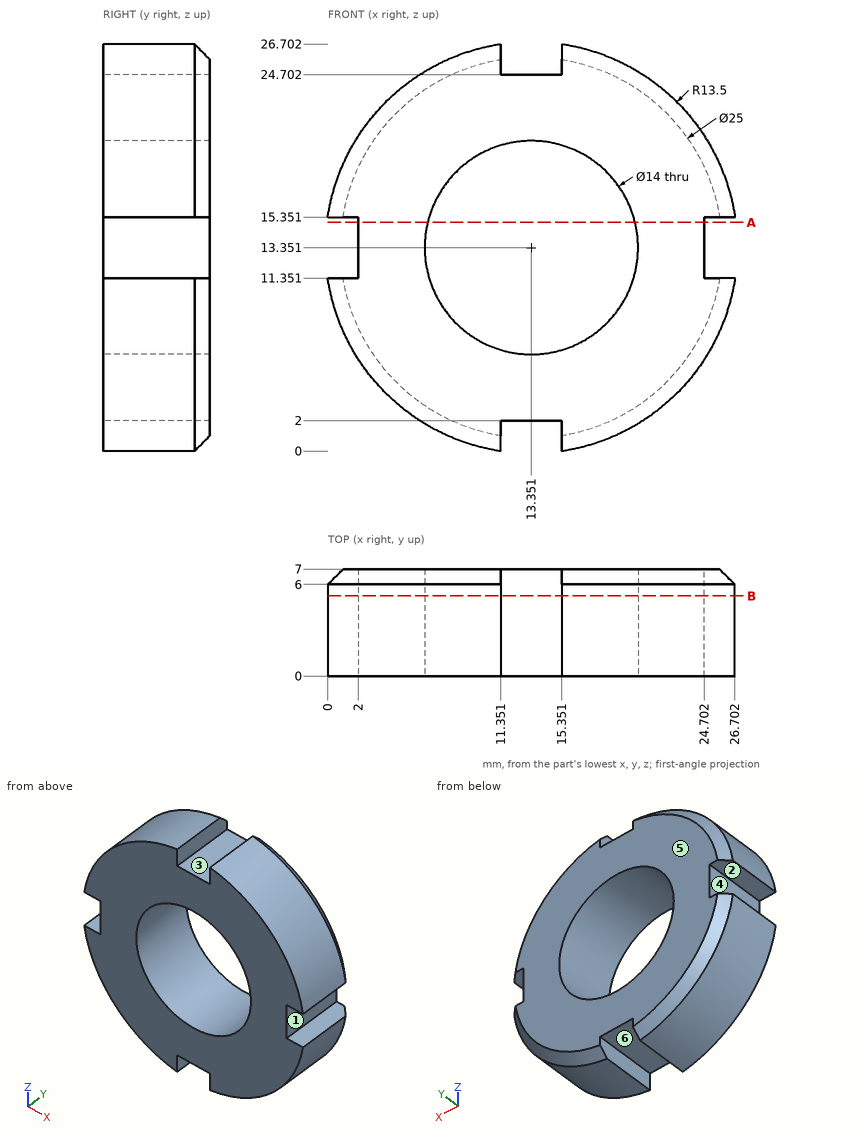
Check sheet for the drawn part. Datum: minimum x, y, z corner. Units: mm. A direction names the side the tool comes from. Round coordinates to 2 decimals unless told otherwise and drop trailing zeros. Loops run counter-clockwise (first coordinate to the right, second up) from the corner with the lowest first, then second, coordinate; pieces in that order, holes last. Notation, with made-up numbers: (70, -12) -> (114, -12) arc R13 cw to (114, 8) -> close; hole circle Ø5 at (84.5, 85.25). An arc over 180 degrees is marked (long way). Put each result on its own line as item: value. Start each with the question number.
1. Draft check along Z on the marked faces 4, 5 and 6. Enter one of: +Z half, -Z half, draft (parallel to the pull), parting line (faces both ways), or undercut.
2. Scan lines: probe 1 along X at (y, z) = (2.75, 12.5); probe 2 along Z at (x, y) = (11.75, 2); probe 3 along X at (y, z) = (2.5, 10) (1 decimal). Record each from-to range of solid material in increasing order.
3. Access from +Z, -Z, +X, -X, +Y, -Y to the whole of each face (thin tool, end or side, straight path). Record for the marked faces 1, 2 and 3.
4. Section check A-A (z = 15). Enter the section's corners in (x, y), plus the area to 3 significant figures.
5. Gauge pin test, flat ends, axial feed: pin 1 (5 mm diameter, centred on x = 9, z = 12.5, fed in from +Y); pin 2 (0.6 mm diameter, centred on y = 5, z = 25.5, fed in from +X); pin 3 (1.2 mm diameter, centred on y = 4.5, z = 14, fed in from +X); pin 4 (1 mm diameter, centred on y = 5, z = 25.5, fed in from -X). Record the tip position at first contact, or that the pin passes through.
6. Section check B-B (y = 5.25). Enter the section's corners in (x, z).
Findings:
1. face 4: undercut
1. face 5: draft
1. face 6: -Z half
2. probe 1: x = 2 to 6.4, 20.3 to 24.7
2. probe 2: z = 2 to 6.54, 20.17 to 24.7
2. probe 3: x = 0.3 to 7.2, 19.5 to 26.4
3. face 1: +X, +Y, -Y
3. face 2: -X, +Y, -Y
3. face 3: +Z, +Y, -Y
4. outline: (2, 0) -> (6.55, 0) -> (6.55, 7) -> (2, 7) -> close; (20.15, 0) -> (24.7, 0) -> (24.7, 7) -> (20.15, 7) -> close
4. area: 63.7 mm^2
5. pin 1: passes through
5. pin 2: stops at x = 19.82
5. pin 3: stops at x = 24.7
5. pin 4: stops at x = 6.53
6. outline: (0, 11.35) arc R13.5 ccw to (11.35, 0) -> (11.35, 2) -> (15.35, 2) -> (15.35, 0) arc R13.5 ccw to (26.7, 11.35) -> (24.7, 11.35) -> (24.7, 15.35) -> (26.7, 15.35) arc R13.5 ccw to (15.35, 26.7) -> (15.35, 24.7) -> (11.35, 24.7) -> (11.35, 26.7) arc R13.5 ccw to (0, 15.35) -> (2, 15.35) -> (2, 11.35) -> close; hole circle Ø14 at (13.35, 13.35)
